from build123d import *

# Parameters (mm, degrees)
SKETCH2_W           = 21
SKETCH2_H           = 14
BOSS_EXTRUDE1_DEPTH = 9
SKETCH3_W           = 15
SKETCH3_H           = 5
CUT_EXTRUDE1_DEPTH  = 5
SKETCH6_W           = 17
SKETCH6_H           = 7
CUT_EXTRUDE3_DEPTH  = 4
SKETCH7_W           = 17
SKETCH7_H           = 5
CUT_EXTRUDE4_DEPTH  = 4
SKETCH8_W           = 1
SKETCH8_H           = 3
CUT_EXTRUDE6_DEPTH  = 4


with BuildPart() as part:
    # Sketch2 → Boss-Extrude1 (new body)
    with BuildSketch(Plane.XY):
        Rectangle(SKETCH2_W, SKETCH2_H)
    extrude(amount=BOSS_EXTRUDE1_DEPTH)

    # Sketch3 → Cut-Extrude1 (cut)
    with BuildSketch(Plane.XY.offset(9)):
        with Locations((0, -2.5)):
            Rectangle(SKETCH3_W, SKETCH3_H)
    extrude(amount=-CUT_EXTRUDE1_DEPTH, mode=Mode.SUBTRACT)

    # Sketch6 → Cut-Extrude3 (cut)
    with BuildSketch(Plane(origin=(0, 7, 0), x_dir=(1, 0, 0), z_dir=(0, 1, 0))):
        with Locations((0, -3.5)):
            Rectangle(SKETCH6_W, SKETCH6_H)
    extrude(amount=-CUT_EXTRUDE3_DEPTH, mode=Mode.SUBTRACT)

    # Sketch7 → Cut-Extrude4 (cut)
    with BuildSketch(Plane(origin=(0, 3, 0), x_dir=(1, 0, 0), z_dir=(0, 1, 0))):
        with Locations((0, -4.5)):
            Rectangle(SKETCH7_W, SKETCH7_H)
    extrude(amount=-CUT_EXTRUDE4_DEPTH, mode=Mode.SUBTRACT)

    # Sketch8 → Cut-Extrude6 (cut)
    with BuildSketch(Plane(origin=(0, -1, 0), x_dir=(1, 0, 0), z_dir=(0, 1, 0))):
        with Locations((-8, -5.5)):
            Rectangle(SKETCH8_W, SKETCH8_H)
        with Locations((8, -5.5)):
            Rectangle(SKETCH8_W, SKETCH8_H)
    extrude(amount=-CUT_EXTRUDE6_DEPTH, mode=Mode.SUBTRACT)


solid = part.part
CAD build for the part. Positions are in the model's coordinates, mm. A direction names the side the tool comes from. Coordinates: 2 decimals unless noted, no trailing zeros. Order: outer loops, then holes, each group sorted by start corner. A loop starts at its lowest first (then second) coordinate and runs counter-clockwise, first axis right, second up. Notation, with made-up numbers: (66, 46) -> (77, 46) arc R12 ccw to (77, 54) -> close; hole circle Ø10 at (65, 3). An arc over 180 degrees is marked (long way). Answer in a Markdown table with one row per item.
1) Which spindle directions (+Z, -Z, +X, -X, +Y, -Y) get a long thin tool onto all of the face, cutting with end or side? Do faces 4 (the face through (8.5, 2, 4)), 5 (the face through (0, 3, 1)), 6 (the face through (0, 0, 8)). Say none if no direction does.
Check values:
| item | result |
|---|---|
| face 4 | +Y |
| face 5 | -Z, +Y |
| face 6 | +Z |
2) Mould opens along Y. For faces 1 (the face through (-0.1, 7, 7.4)), 2 (the face through (0, -5, 7)), 3 (the face through (0, -3, 4)) say: pulls with the +Y half, pulls with the -Y half, needs draft (parallel to the pull), parting line crosses it, or undercut.
Check values:
| item | result |
|---|---|
| face 1 | pulls with the +Y half |
| face 2 | undercut |
| face 3 | needs draft |
3) Band-saw the part on B-B (z = 7.75). List the corners of the cut face in (x, y).
Check values:
| item | result |
|---|---|
| outline | (-10.5, -7) -> (10.5, -7) -> (10.5, 7) -> (-10.5, 7) -> close; hole (-7.5, -5) -> (7.5, -5) -> (7.5, 0) -> (-7.5, 0) -> close |
4) Band-saw the part on A-A (y = 1.5). List the corners of the cut face in (x, z), and give its area (3 significant figures).
Check values:
| item | result |
|---|---|
| outline | (-10.5, 0) -> (10.5, 0) -> (10.5, 9) -> (-10.5, 9) -> close; hole (-8.5, 2) -> (8.5, 2) -> (8.5, 7) -> (-8.5, 7) -> close |
| area | 104 mm2 |
5) Band-saw the part on D-D (x = 7.75). List the corners of the cut face in (y, z).
Check values:
| item | result |
|---|---|
| outline | (-7, 0) -> (3, 0) -> (3, 2) -> (-1, 2) -> (-1, 4) -> (-5, 4) -> (-5, 7) -> (7, 7) -> (7, 9) -> (-7, 9) -> close |
6) Drill centre lines: line 1 (Z direction, x = 8, y = 1.75); line 2 (X direction, y = 5.5, z = 5.5); line 3 (Y direction, x = 3, z = 8). Where is each one in solid material? Low to high.
Check values:
| item | result |
|---|---|
| line 1 | 0 to 2, 7 to 9 |
| line 2 | -10.5 to -8.5, 8.5 to 10.5 |
| line 3 | -7 to -5, 0 to 7 |
7) Flat gauge pins, fed straight in: P1, Ø1.2, axis at x = -0.5, y = -3.5, coming from the +Z side; P2, Ø0.6, axis at x = -2, z = 1, coming from the +Y side. Where does each tip first touch, or does it go through?
Check values:
| item | result |
|---|---|
| P1 | z = 4 |
| P2 | y = 3 |
8) Band-saw the part on C-C (x = -2.25). List the corners of the cut face in (y, z), and give its area (3 significant figures).
Check values:
| item | result |
|---|---|
| outline | (-7, 0) -> (3, 0) -> (3, 2) -> (-1, 2) -> (-1, 4) -> (-5, 4) -> (-5, 9) -> (-7, 9) -> close; (0, 7) -> (7, 7) -> (7, 9) -> (0, 9) -> close |
| area | 56.0 mm2 |
